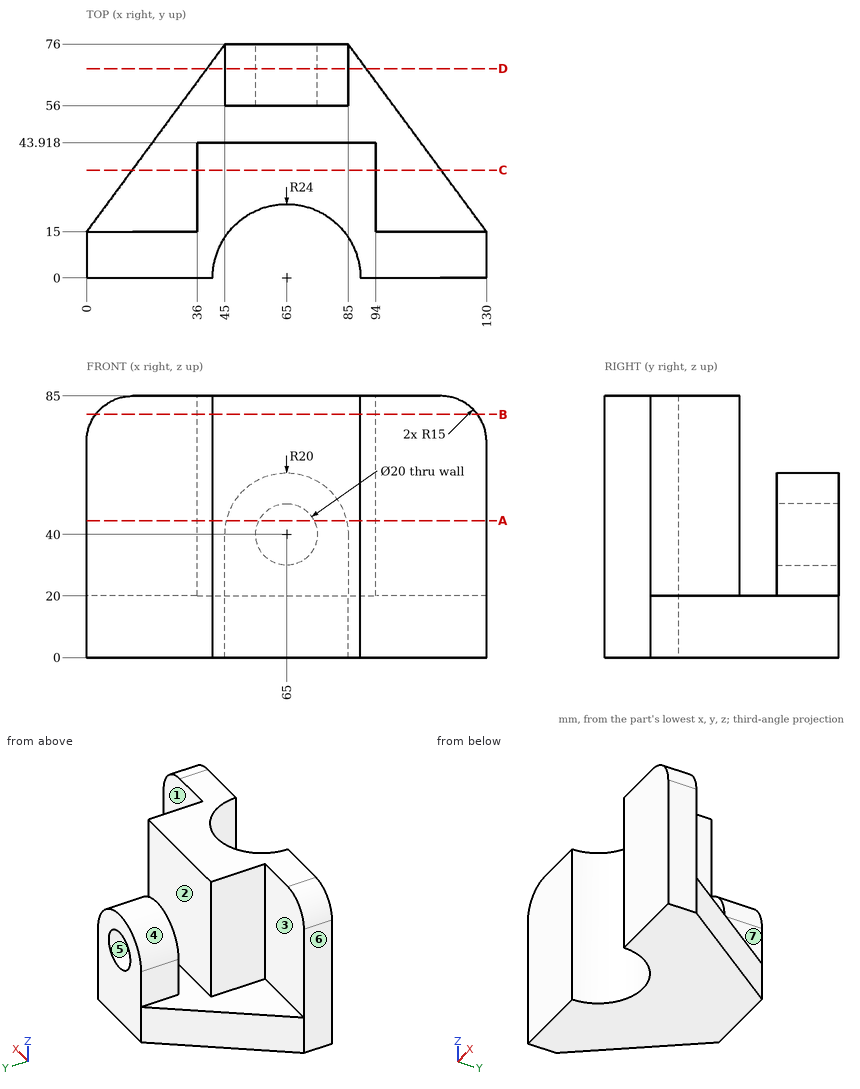
The figure shows three views and two pictorial views of one solid part (mm, origin at its lowest corner). Answer the questions. A direction names the side the tool comes from. Give positions to 0.01 mm unless a question says otherwise; leave off trailing zeros. Write each loop counter-clockwise with the first axis right and the second up, starting at its lowest first coordinate (ties: lowest second). Pieces come first, ordered by that corner, then holes. Notation, with made-up numbers: (51, 21.5) -> (85, 21.5) arc R28 cw to (85, 57.5) -> close; hole circle Ø9 at (53, 16). An arc over 180 degrees is marked (long way). Use one line per item in the form item = value.
1) Section C-C on y = 35 is taken. Write down the section's boundary in (x, z).
Result:
outline = (14.75, 0) -> (115.25, 0) -> (115.25, 20) -> (94, 20) -> (94, 85) -> (36, 85) -> (36, 20) -> (14.75, 20) -> close
2) Section B-B on z = 79 is taken. Write down the section's boundary in (x, y).
Result:
outline = (3, 0) -> (41, 0) arc R24 cw to (89, 0) -> (127, 0) -> (127, 15) -> (94, 15) -> (94, 43.92) -> (36, 43.92) -> (36, 15) -> (3, 15) -> close
3) Straight lines are drawn through the part: probe 1 along X at (y, z) = (67, 40); probe 2 along Y at (x, z) = (6, 35); probe 3 along Y at (x, z) = (91, 68). For each, find the intervals that lie inside material, in ascending order.
Result:
probe_1 = 45 to 55, 75 to 85
probe_2 = 0 to 15
probe_3 = 0 to 43.92
4) A tool of negligible diameter and unlimited length cuts with its end or side. For the marked faces 1, 2, 3 and 4, from which of +Z, -Z, +X, -X, +Y, -Y can it reach the whole face along a straight path? Write none if from no direction.
Result:
face_1 = +Z, +X, +Y
face_2 = +Z, +X, -X
face_3 = +Z, -X, +Y
face_4 = +Z, +Y
5) For a pull along X with two mould halves and no side action, classify the marked faces 5, 6 and 7 as +X half, -X half, draft (parallel to the pull), parting line (faces both ways), or undercut.
Result:
face_5 = undercut
face_6 = -X half
face_7 = +X half
6) Section D-D on y = 68 is taken. Write down the section's boundary in (x, z).
Result:
outline = (39.1, 0) -> (90.9, 0) -> (90.9, 20) -> (85, 20) -> (85, 40) arc R20 ccw to (45, 40) -> (45, 20) -> (39.1, 20) -> close; hole circle Ø20 at (65, 40)
7) Each of these flat-tipped pins is pushed along its axis until it touches: P1, Ø2, axis at y = 63, z = 46.5, coming from the +X side; P2, Ø11, axis at x = 22, z = 37, coming from the +Y side; P3, Ø22, axis at y = 68, z = 32, coming from the +X side; P4, Ø10, axis at y = 54, z = 69, coming from the -X side. Where does it stop, or does it pass through?
Result:
P1 = 84.23
P2 = 15
P3 = 85
P4 = through
8) Section A-A on z = 44.5 is taken. Write down the section's boundary in (x, y).
Result:
outline = (0, 0) -> (41, 0) arc R24 cw to (89, 0) -> (130, 0) -> (130, 15) -> (94, 15) -> (94, 43.92) -> (36, 43.92) -> (36, 15) -> (0, 15) -> close; (45.51, 56) -> (56.07, 56) -> (56.07, 76) -> (45.51, 76) -> close; (73.93, 56) -> (84.49, 56) -> (84.49, 76) -> (73.93, 76) -> close
